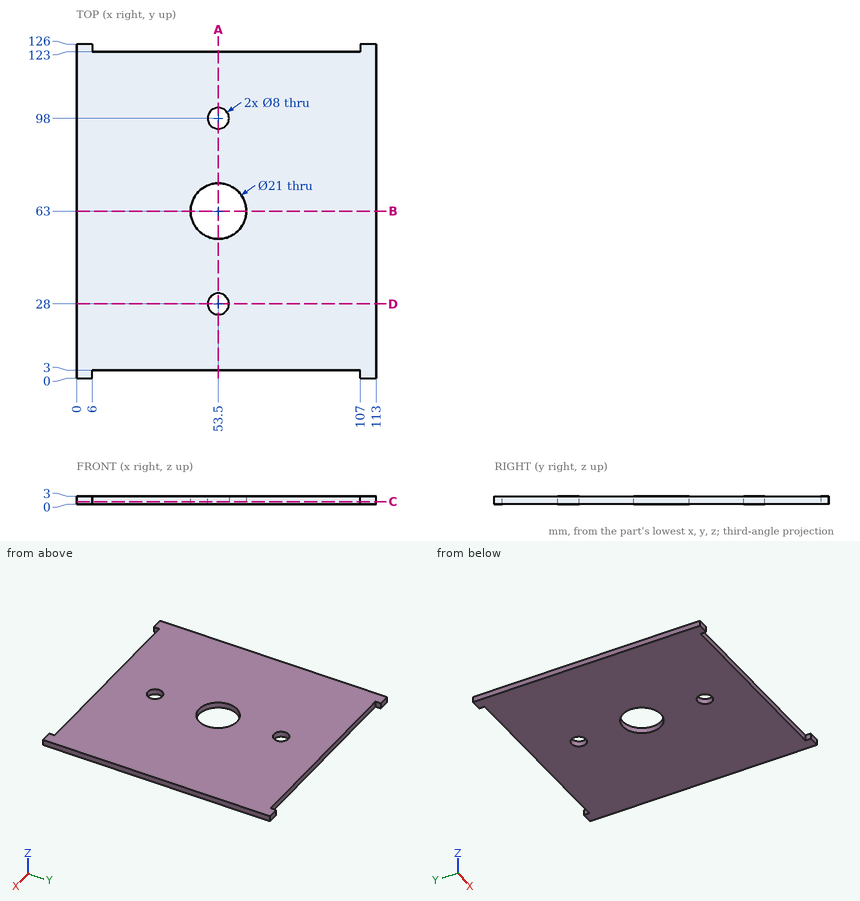
Check sheet for the drawn part. Datum: minimum x, y, z corner. Units: mm. Give positions to 0.01 mm unless a question says otherwise; leave off trailing zeros. Loops run counter-clockwise (first coordinate to the right, second up) from the corner with the lowest first, then second, coordinate; pieces in that order, holes last.
1) Thickness scan on line 1 along Y through (x, z) = (53.5, 2.45); line 2 along X through (y, z) = (63, 1.5); line 3 along Y through (x, z) = (27, 0.7). Record the ranges inside material, lowest first.
2) Sectioned sample at C-C, the plane z = 1. Enter the section's corners in (x, y).
3) Sectioned sample at D-D, the plane y = 28. Enter the section's corners in (x, z).
4) Sectioned sample at A-A, the plane x = 53.5. Enter the section's corners in (y, z).
5) Depth check by flat-ended pin: pin 1 Ø6.5 at (x, y) = (53.5, 98) entering from +Z; pin 2 Ø0.9 at (x, z) = (44.5, 1.5) entering from -Y; pin 3 Ø1.5 at (x, z) = (36, 2) entering from +Y. Enter the tip coordinate at first touch or a pass-through.
6) Sectioned sample at B-B, the plane y = 63. Enter the section's corners in (x, z).
Answers:
1. line 1: y = 3 to 24, 32 to 52.5, 73.5 to 94, 102 to 123
1. line 2: x = 0 to 43, 64 to 113
1. line 3: y = 3 to 123
2. outline: (0, 0) - (6, 0) - (6, 3) - (107, 3) - (107, 0) - (113, 0) - (113, 126) - (107, 126) - (107, 123) - (6, 123) - (6, 126) - (0, 126) - close; hole circle Ø21 at (53.5, 63); hole circle Ø8 at (53.5, 28); hole circle Ø8 at (53.5, 98)
3. outline: (0, 0) - (49.5, 0) - (49.5, 3) - (0, 3) - close; (57.5, 0) - (113, 0) - (113, 3) - (57.5, 3) - close
4. outline: (3, 0) - (24, 0) - (24, 3) - (3, 3) - close; (32, 0) - (52.5, 0) - (52.5, 3) - (32, 3) - close; (73.5, 0) - (94, 0) - (94, 3) - (73.5, 3) - close; (102, 0) - (123, 0) - (123, 3) - (102, 3) - close
5. pin 1: passes through
5. pin 2: stops at y = 3
5. pin 3: stops at y = 123
6. outline: (0, 0) - (43, 0) - (43, 3) - (0, 3) - close; (64, 0) - (113, 0) - (113, 3) - (64, 3) - close
